Could you check a few things on this model? Use its own coordinates, in mm. A direction names the side the tool comes from. Give positions to 0.01 mm unless a question says otherwise; leave off trailing zeros. Write each loop counter-clockwise with the first axis right and the second up, starting at its lowest first coordinate (ties: lowest second). Pieces come first, ordered by that corner, then holes. Notation, with made-up numbers: M 77.5,38 L 97.5,38 A31 cw 97.5,76 Z; hole C 47,50.25 d11. An arc over 180 degrees is marked long. Use one line per item in the form item = value.
from build123d import *

# Parameters (mm, degrees)
F0_R     = 4.65
F0_R_2   = 2.55
F1_DEPTH = 1.4
F2_DEPTH = 9
F3_DEPTH = 19.3
F4_DEPTH = 16.7
F0_R_3   = 1.4
F5_DEPTH = 1.1


with BuildPart() as f1:
    # F0 (on Top) → F1 (new body)
    with BuildSketch(Plane.XY):
        with Locations((0, 8.25)):
            Circle(F0_R)
        with Locations((0, 8.25)):
            Circle(F0_R_2, mode=Mode.SUBTRACT)
    extrude(amount=F1_DEPTH)

    # F0 (on Top) → F2 (join)
    with BuildSketch(Plane.XY):
        with Locations((0, 8.25)):
            Circle(F0_R_2)
    extrude(amount=F2_DEPTH)

    # F0 (on Top) → F3 (join)
    with BuildSketch(Plane.XY):
        with BuildLine():
            ThreePointArc((-7.35, -12.0327677614), (0, -14.1), (7.35, -12.0327677614))
            Line((7.35, -12.0327677614), (-7.35, -12.0327677614))
        make_face()
        with BuildLine():
            Line((13.6193795747, -3.65), (13.6193795747, 3.65))
            ThreePointArc((13.6193795747, 3.65), (0, 14.1), (-13.6193795747, 3.65))
            ThreePointArc((-13.6193795747, 3.65), (-14.1, 0), (-13.6193795747, -3.65))
            ThreePointArc((-13.6193795747, -3.65), (-11.2914312101, -8.4447368951), (-7.35, -12.0327677614))
            Line((-7.35, -12.0327677614), (7.35, -12.0327677614))
            ThreePointArc((7.35, -12.0327677614), (11.2914312101, -8.4447368951), (13.6193795747, -3.65))
        make_face()
        with Locations((0, 8.25)):
            Circle(F0_R, mode=Mode.SUBTRACT)
        with Locations((0, 8.25)):
            Circle(F0_R)
        with Locations((0, 8.25)):
            Circle(F0_R_2, mode=Mode.SUBTRACT)
        with Locations((0, 8.25)):
            Circle(F0_R_2)
        with BuildLine():
            ThreePointArc((13.6193795747, -3.65), (13.9793285247, -1.8407536495), (14.1, 0))
            ThreePointArc((14.1, 0), (13.9793285247, 1.8407536495), (13.6193795747, 3.65))
            Line((13.6193795747, 3.65), (13.6193795747, -3.65))
        make_face()
    extrude(amount=-F3_DEPTH)

    # F0 (on Top) → F4 (join)
    with BuildSketch(Plane.XY):
        with BuildLine():
            Line((7.35, -16.2327677614), (7.35, -12.0327677614))
            ThreePointArc((7.35, -12.0327677614), (0, -14.1), (-7.35, -12.0327677614))
            Line((-7.35, -12.0327677614), (-7.35, -16.2327677614))
            Line((-7.35, -16.2327677614), (7.35, -16.2327677614))
        make_face()
    extrude(amount=-F4_DEPTH)

    # F0 (on Top) → F5 (join)
    with BuildSketch(Plane.XY):
        with BuildLine():
            ThreePointArc((-13.6193795747, -3.65), (-14.1, 0), (-13.6193795747, 3.65))
            Line((-13.6193795747, 3.65), (-17.4693795747, 3.65))
            ThreePointArc((-17.4693795747, 3.65), (-20.050319326, 2.5809397513), (-21.1193795747, 0))
            ThreePointArc((-21.1193795747, 0), (-20.050319326, -2.5809397513), (-17.4693795747, -3.65))
            Line((-17.4693795747, -3.65), (-13.6193795747, -3.65))
        make_face()
        with Locations((-17.4, 0)):
            Circle(F0_R_3, mode=Mode.SUBTRACT)
        with BuildLine():
            ThreePointArc((13.6193795747, 3.65), (13.9793285247, 1.8407536495), (14.1, 0))
            ThreePointArc((14.1, 0), (13.9793285247, -1.8407536495), (13.6193795747, -3.65))
            Line((13.6193795747, -3.65), (17.4693795747, -3.65))
            ThreePointArc((17.4693795747, -3.65), (20.050319326, -2.5809397513), (21.1193795747, 0))
            ThreePointArc((21.1193795747, 0), (20.050319326, 2.5809397513), (17.4693795747, 3.65))
            Line((17.4693795747, 3.65), (13.6193795747, 3.65))
        make_face()
        with Locations((17.4, 0)):
            Circle(F0_R_3, mode=Mode.SUBTRACT)
    extrude(amount=-F5_DEPTH)


solid = f1.part
1) I want a section at C-C, the plane y = 3. Please give me the cut outline in (x, z).
Checked values:
outline = M -19.55,-1.1 L -13.78,-1.1 L -13.78,-19.3 L 13.78,-19.3 L 13.78,-1.1 L 19.55,-1.1 L 19.55,0 L -19.55,0 Z
2) I want a section at B-B, the plane x = 0. Please give me the cut outline in (y, z), plus the area to 3 significant figures.
Checked values:
outline = M -16.23,-16.7 L -14.1,-16.7 L -14.1,-19.3 L 14.1,-19.3 L 14.1,0 L 12.9,0 L 12.9,1.4 L 10.8,1.4 L 10.8,9 L 5.7,9 L 5.7,1.4 L 3.6,1.4 L 3.6,0 L -16.23,0 Z
area = 632 mm2
3) For pin 1 Ø1 at (x, y) = (-1.5, -3) entering from +Z; pin 2 Ø1.3 at (y, z) = (-15, -8) entering from -X; pin 3 Ø12 at (x, z) = (-15, -2) entering from +Y, each with a flat end and sliding along its axis, tell me the tip position at first contact or that it passes through.
Checked values:
pin_1 = 0
pin_2 = -7.35
pin_3 = 10.85
4) I want a section at A-A, the plane z = -17.25. Please give me the cut outline in (x, y).
Checked values:
outline = C 0,0 d28.2
5) If I drill on L1, parallel to Y at x = -17.4, z = -0.8; L2, parallel to Z at x = 4.5, y = 5.5; L3, parallel to Z at x = -1, y = 11.5, over which ranges is the centre line in solid material (lowest first)?
Checked values:
L1 = -3.65 to -1.4, 1.4 to 3.65
L2 = -19.3 to 0
L3 = -19.3 to 1.4
6) Thinking about a two-plate mould opening in X: for faces 6 (the cylindrical face through (-18.8, 0.06, -0.54)), 7 (the cylindrical face through (-0.55, 5.76, 5.15)), 8 (the flat face through (7.35, -14, -8)), which applies, released by +X, released by -X, zero draft, split by the parting line, or undercut?
Checked values:
face_6 = undercut
face_7 = split by the parting line
face_8 = released by +X
7) For faces 1 (the flat face through (15.6, 3.65, -0.5)), 2 (the cylindrical face through (-1.01, 3.71, 0.69)), 3 (the flat face through (15.5, -3.65, -0.5)), 4 (the flat face through (-15.5, 3.65, -0.5)), 5 (the flat face through (-15.6, -3.65, -0.5)), which set-ups out of +Z, -Z, +X, -X, +Y, -Y let a thin tool reach every point of the face, with its end or its side?
Checked values:
face_1 = +Z, -Z, +X, +Y
face_2 = +Z
face_3 = +Z, -Z, +X, -Y
face_4 = +Z, -Z, -X, +Y
face_5 = +Z, -Z, -X, -Y
8) I want a section at D-D, the plane z = 0.5. Please give me the cut outline in (x, y).
Checked values:
outline = C 0,8.25 d9.3
